Part model, mm, in its own coordinate system. A direction names the side the tool comes from. Coordinates: 2 decimals unless noted, no trailing zeros. Order: outer loops, then holes, each group sorted by start corner. A loop starts at its lowest first (then second) coordinate and runs counter-clockwise, first axis right, second up.
```python
from build123d import *

# Parameters (mm, degrees)
F1_DEPTH = 15
F3_D     = 3.8
F4_R     = 1.9
F5_DEPTH = 2.7


with BuildPart() as f1:
    # F0 (on Front) → F1 (new body)
    with BuildSketch(Plane.XZ):
        Polygon((0, 7), (0, 0), (6.2, 0), (8.6, 2.4), (8.6, 4.4), (5, 4.4), (5, 7), align=None)
        Polygon((-8.6, 4.4), (-8.6, 2.4), (-6.2, 0), (0, 0), (0, 7), (-5, 7), (-5, 4.4), align=None)
    extrude(amount=F1_DEPTH)

    # F3 (through all)
    with Locations(Plane.XY.offset(7)):
        with Locations((0, -7.5)):
            Hole(F3_D / 2)

    # F4 (on face) → F5 (cut)
    with BuildSketch(Plane(origin=(0, 0, 0), x_dir=(1, 0, 0), z_dir=(0, 0, -1))):
        Polygon((-3, 5.7679491924), (0, 4.0358983849), (3, 5.7679491924), (3, 9.2320508076), (0, 10.9641016151), (-3, 9.2320508076), align=None)
        with Locations((0, 7.5)):
            Circle(F4_R, mode=Mode.SUBTRACT)
    extrude(amount=-F5_DEPTH, mode=Mode.SUBTRACT)


solid = f1.part
```
(1) Slice it at C-C, the plane y = -11.5. Give the cut face in (x, z).
(2) Tool access for faces 1 (the face through (-7, -7, 4.4)), 2 (the face through (7, -7, 4.4)), 3 (the face through (-7.4, -7.4, 1.2)), 4 (the face through (1.2, -5.7, 7)), 5 (the face through (-1.4, -6, 2.7)): list every direction of +Z, -Z, +X, -X, +Y, -Y with a clear straight run to the whole face (end or side of a thin tool).
(3) Slice it at B-B, the plane z = 1.5. Give the cut face in (x, y), then the cut area to 3 significant figures.
(4) Slice it at A-A, the plane y = -7.5. Give the cut face in (x, z).
(5) Drop flat-ended pins along their axis: pin 1 (5 mm diameter, centred on x = 0, y = -7.5, fed in from -Z); pin 2 (2 mm diameter, centred on y = -8, z = 5.5, fed in from -X); pin 3 (1.3 mm diameter, centred on y = -10, z = 5.5, fed in from +X). Give the stop position or say it passes through.
(6) Slice it at D-D, the plane z = 6.25. Give the cut face in (x, y), then the cut area to 3 significant figures.
(7) Probe line 1 (X direction, y = -7.5, z = 6); line 2 (Y direction, x = 0, z = 5.75); line 3 (X direction, y = -6.5, z = 2.5). List the from-to ranges inside material, lowest first.
Here are the results:
1. outline: (-8.6, 2.4) - (-6.2, 0) - (6.2, 0) - (8.6, 2.4) - (8.6, 4.4) - (5, 4.4) - (5, 7) - (-5, 7) - (-5, 4.4) - (-8.6, 4.4) - close
2. face 1: +Z, -X, +Y, -Y
2. face 2: +Z, +X, +Y, -Y
2. face 3: -Z, -X, +Y, -Y
2. face 4: +Z, +X, -X, +Y, -Y
2. face 5: -Z
3. outline: (-7.7, -15) - (7.7, -15) - (7.7, 0) - (-7.7, 0) - close; hole (-3, -9.23) - (0, -10.96) - (3, -9.23) - (3, -5.77) - (0, -4.04) - (-3, -5.77) - close
3. area: 200 mm2
4. outline: (-8.6, 2.4) - (-6.2, 0) - (-3, 0) - (-3, 2.7) - (-1.9, 2.7) - (-1.9, 7) - (-5, 7) - (-5, 4.4) - (-8.6, 4.4) - close; (1.9, 2.7) - (3, 2.7) - (3, 0) - (6.2, 0) - (8.6, 2.4) - (8.6, 4.4) - (5, 4.4) - (5, 7) - (1.9, 7) - close
5. pin 1: stops at z = 2.7
5. pin 2: stops at x = -5
5. pin 3: stops at x = 5
6. outline: (-5, -15) - (5, -15) - (5, 0) - (-5, 0) - close; hole circle Ø3.8 at (0, -7.5)
6. area: 139 mm2
7. line 1: x = -5 to -1.9, 1.9 to 5
7. line 2: y = -15 to -9.4, -5.6 to 0
7. line 3: x = -8.6 to -3, 3 to 8.6
